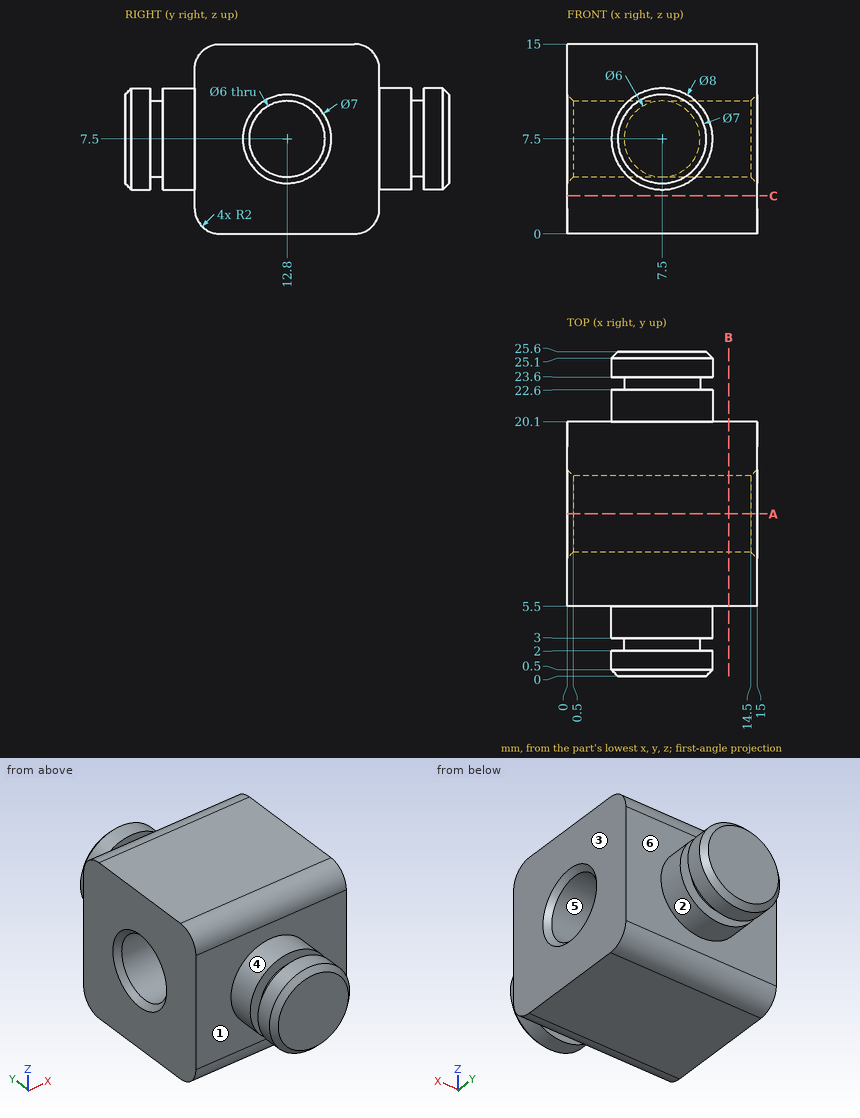
Can you work these out from the drawing? Everything is in mm from the part's minimum corner. A direction names the side the tool comes from. Give positions to 0.01 mm unless a question says otherwise; leave off trailing zeros. Order: outer loops, then holes, each group sorted by start corner. A loop starts at its lowest first (then second) coordinate and runs counter-clockwise, first axis right, second up.
Item 1: If we section it at A-A, the plane y = 12.8: Write out the boundary of the cut face in (x, z).
Item 2: If we section it at C-C, the plane z = 3: Write out the boundary of the cut face in (x, y), plus the area to 3 significant figures.
Item 3: I need wall thicknesses on line 1 (Z direction, x = 9.25, y = 12.8); line 2 (Y direction, x = 10.75, z = 8.5); line 3 (Y direction, x = 10, z = 4). Which ranges of each line are inside material? Lowest first, please.
Item 4: If we section it at B-B, the plane x = 12.75: Write out the boundary of the cut face in (y, z), plus the area to 3 significant figures.
Item 5: If we mould it in two halves opening along Z, with no side actions, what happens to the marked faces 4, 5 and 6? For each: pulls with the +Z half, pulls with the -Z half, needs draft (parallel to the pull), parting line crosses it, or undercut.
Item 6: I'm going to push flat-ended pins straight in: pin 1 (1.5 mm diameter, centred on x = 6, y = 21.5, fed in from +Z); pin 2 (2 mm diameter, centred on x = 12.5, z = 9, fed in from -Y). Where does each tip first touch, or does it pass through?
Item 7: For the marked faces 1, 2 and 3, which set-ups out of +Z, -Z, +X, -X, +Y, -Y let a thin tool reach every point of the face, with its end or its side?
Values:
1. outline: (0, 0) - (15, 0) - (15, 4) - (14.5, 4.5) - (0.5, 4.5) - (0, 4) - close; (0, 11) - (0.5, 10.5) - (14.5, 10.5) - (15, 11) - (15, 15) - (0, 15) - close
2. outline: (0, 5.5) - (15, 5.5) - (15, 20.1) - (0, 20.1) - close
2. area: 219 mm2
3. line 1: z = 0 to 4.5, 10.5 to 15
3. line 2: y = 0 to 2, 3 to 9.97, 15.63 to 22.6, 23.6 to 25.6
3. line 3: y = 5.5 to 20.1
4. outline: (5.5, 2) arc R2 ccw to (7.5, 0) - (18.1, 0) arc R2 ccw to (20.1, 2) - (20.1, 13) arc R2 ccw to (18.1, 15) - (7.5, 15) arc R2 ccw to (5.5, 13) - close; hole circle Ø6 at (12.8, 7.5)
4. area: 187 mm2
5. face 4: parting line crosses it
5. face 5: undercut
5. face 6: needs draft
6. pin 1: stops at z = 11.43
6. pin 2: stops at y = 5.5
7. face 1: -Y
7. face 2: +Y
7. face 3: +Z, -Z, +X, +Y, -Y
